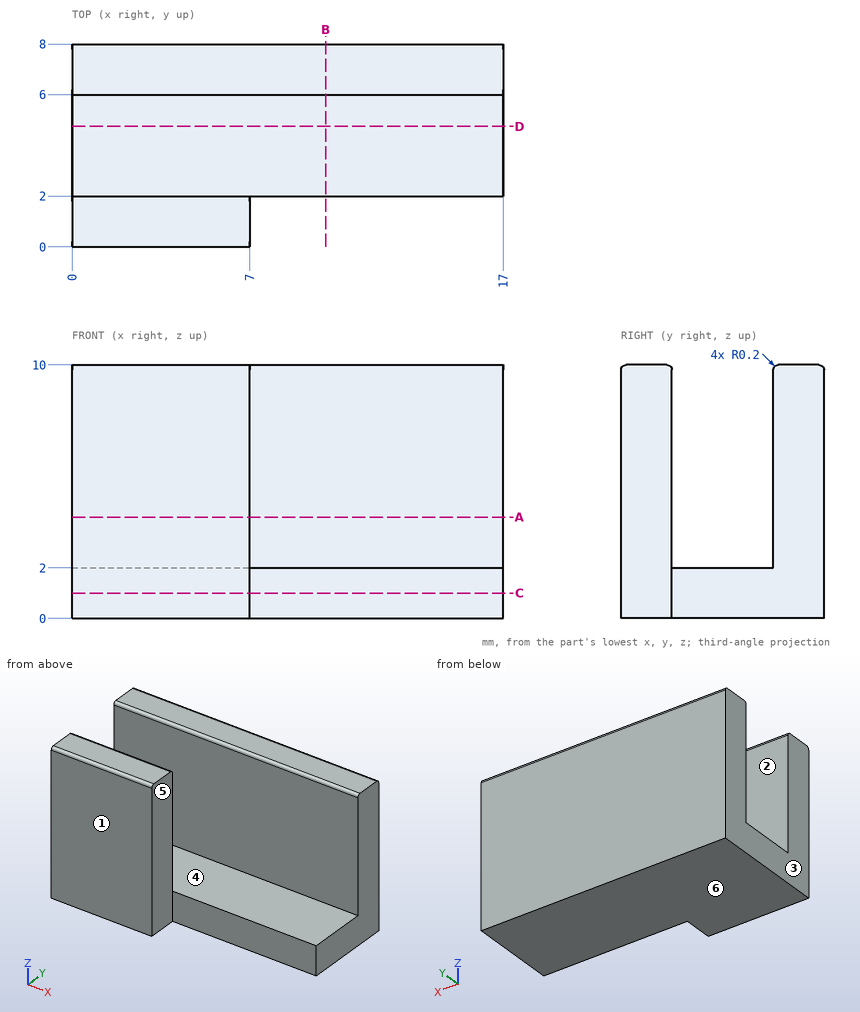
Part print with two shaded views. Sizes in mm from the minimum x, y, z corner. A direction names the side the tool comes from. Coordinates: 2 decimals unless noted, no trailing zeros. Loops run counter-clockwise (first coordinate to the right, second up) from the corner with the lowest first, then second, coordinate; pieces in that order, holes last. Notation, with made-up numbers: (-15, 50.5) -> (8, 50.5) arc R23 cw to (8, 82.5) -> close; hole circle Ø6 at (-33, 68.25). An arc over 180 degrees is marked (long way). Answer as a JSON object with one key per item and string values.
Q1. Pull direction Y, two halves, no side cores. Call the marked faces 1, 2 and 3: released by +Y, released by -Y, zero draft, split by the parting line, or undercut.
Report:
{"face 1": "released by -Y", "face 2": "undercut", "face 3": "zero draft"}
Q2. 3-axis set-ups, long thin cutter, end or side, ignore diameter. For the marked faces 4, 5 and 6: which of +Z, -Z, +X, -X, +Y, -Y reach the whole face in a straight line?
Report:
{"face 4": "+Z, +X, -X", "face 5": "+Z, -Z, +X, -Y", "face 6": "-Z, +X, -X, +Y, -Y"}
Q3. Flat gauge pins, fed straight in: P1, Ø1.6, axis at y = 0.5, z = 7, coming from the +X side; P2, Ø1.6, axis at x = 13.5, z = 1, coming from the -Y side; P3, Ø4, axis at x = 10.5, z = 7, coming from the -Y side. Where does each tip first touch, or does it go through?
Report:
{"P1": "stops at x = 7", "P2": "stops at y = 2", "P3": "stops at y = 6"}
Q4. Cut at C-C (z = 1). List the corners of the cut face in (x, y), and give its area (3 significant figures).
Report:
{"outline": "(0, 0) -> (7, 0) -> (7, 2) -> (17, 2) -> (17, 8) -> (0, 8) -> close", "area": "116 mm2"}
Q5. Cut at B-B (x = 10). List the corners of the cut face in (y, z).
Report:
{"outline": "(2, 0) -> (8, 0) -> (8, 9.8) arc R0.2 ccw to (7.8, 10) -> (6.2, 10) arc R0.2 ccw to (6, 9.8) -> (6, 2) -> (2, 2) -> close"}
Q6. Probe probe 1 along Y at (x, z) = (3, 7.75); probe 2 along Z at (x, y) = (8, 3.5); probe 3 along X at (y, z) = (0.75, 1.25). List the from-to ranges inside material, lowest first.
Report:
{"probe 1": "y = 0 to 2, 6 to 8", "probe 2": "z = 0 to 2", "probe 3": "x = 0 to 7"}
Q7. Cut at A-A (z = 4). List the corners of the cut face in (x, y).
Report:
{"outline": "(0, 0) -> (7, 0) -> (7, 2) -> (0, 2) -> close; (0, 6) -> (17, 6) -> (17, 8) -> (0, 8) -> close"}
Q8. Cut at D-D (y = 4.75). List the corners of the cut face in (x, z), and give its area (3 significant figures).
Report:
{"outline": "(0, 0) -> (17, 0) -> (17, 2) -> (0, 2) -> close", "area": "34.0 mm2"}
